```python
from build123d import *

# Parameters (mm, degrees)
CUT_EXTRUDE1_DEPTH      = 8.470943715
CUT_EXTRUDE1_DEPTH_BACK = 8.470943715
SKETCH3_OUTSIDE_W       = 10.214
SKETCH3_OUTSIDE_H       = 10.214
SKETCH3_OUTSIDE_W_2     = 4
SKETCH3_OUTSIDE_H_2     = 5
CUT_EXTRUDE2_DEPTH      = 7.641159537
CUT_EXTRUDE2_DEPTH_BACK = 7.641159537
SKETCH4_OUTSIDE_W       = 9.868
SKETCH4_OUTSIDE_H       = 8.768
SKETCH4_OUTSIDE_W_2     = 5
SKETCH4_OUTSIDE_H_2     = 5
SKETCH5_R               = 0.75
BOSS_EXTRUDE1_DEPTH     = 1.5
SKETCH6_R               = 1.5
BOSS_EXTRUDE2_DEPTH     = 2


with BuildPart() as part:
    # Sketch2 → Revolve3 (revolve)
    with BuildSketch(Plane(origin=(0, 0, 0), x_dir=(0, 0, -1), z_dir=(1, 0, 0))):
        with BuildLine():
            Line((0, 0), (0, 6.1))
            ThreePointArc((0, 6.1), (3.05, 3.05), (0, 0))
        make_face()
    revolve(axis=Axis((0, 0, 0), (0, 1, 0)))

    # Sketch3 outside → Cut-Extrude1 (cut, two sides: drawn at the far end of the back side and taken through both)
    with BuildSketch(Plane(origin=(0, 0, 0), x_dir=(0, 0, -1), z_dir=(1, 0, 0)).offset(-CUT_EXTRUDE1_DEPTH_BACK)):
        with Locations((0, 3.05)):
            Rectangle(SKETCH3_OUTSIDE_W, SKETCH3_OUTSIDE_H)
        with Locations((0, 3.05)):
            Rectangle(SKETCH3_OUTSIDE_W_2, SKETCH3_OUTSIDE_H_2, mode=Mode.SUBTRACT)
    extrude(amount=CUT_EXTRUDE1_DEPTH + CUT_EXTRUDE1_DEPTH_BACK, mode=Mode.SUBTRACT)

    # Sketch4 outside → Cut-Extrude2 (cut, two sides: drawn at the far end of the back side and taken through both)
    with BuildSketch(Plane.XY.offset(-CUT_EXTRUDE2_DEPTH_BACK)):
        with Locations((0, 3.05)):
            Rectangle(SKETCH4_OUTSIDE_W, SKETCH4_OUTSIDE_H)
        with Locations((0, 3.05)):
            Rectangle(SKETCH4_OUTSIDE_W_2, SKETCH4_OUTSIDE_H_2, mode=Mode.SUBTRACT)
    extrude(amount=CUT_EXTRUDE2_DEPTH + CUT_EXTRUDE2_DEPTH_BACK, mode=Mode.SUBTRACT)

    # Sketch5 → Boss-Extrude1 (add)
    with BuildSketch(Plane(origin=(2.5, 0, 0), x_dir=(0, 0, -1), z_dir=(1, 0, 0))):
        with Locations((0, 3.05)):
            Circle(SKETCH5_R)
    boss_extrude1 = extrude(amount=BOSS_EXTRUDE1_DEPTH)

    # Mirror1: Boss-Extrude1 across plane
    add(boss_extrude1.mirror(Plane(origin=(0, 0, 0), x_dir=(0, 0, 1), z_dir=(1, 0, 0))))

    # Sketch6 → Boss-Extrude2 (add)
    with BuildSketch(Plane(origin=(0, 0, -2), x_dir=(-1, 0, 0), z_dir=(0, 0, -1))):
        with Locations(Location((0, 3.05, 0), (0, 0, 90))):
            Circle(SKETCH6_R)
    boss_extrude2 = extrude(amount=BOSS_EXTRUDE2_DEPTH)

    # Mirror2: Boss-Extrude2 across plane
    add(boss_extrude2.mirror(Plane.XY))


solid = part.part
```
Design review of the part built by this model. Coordinates are the model's own, in mm. A direction names the side the tool comes from. Give positions to 0.01 mm unless a question says otherwise; leave off trailing zeros. Write each loop counter-clockwise with the first axis right and the second up, starting at its lowest first coordinate (ties: lowest second). Pieces come first, ordered by that corner, then holes. Notation, with made-up numbers: (75, -37) - (114, -37) arc R14 cw to (114, -30) - close; hole circle Ø8 at (-30.5, 22). An arc over 180 degrees is marked (long way). Return JSON: item names as keys, results as strings. Group by question number.
(1) We need section A-A, the plane y = 3.05. Give the boundary of the cut face in (x, z), then the cut area to 3 significant figures.
(2) Insertion check: pin 1 (1.5 mm diameter, centred on y = 4.5, z = 2, fed in from +X); pin 2 (1 mm diameter, centred on y = 4.5, z = 2, fed in from +X); pin 3 (1.5 mm diameter, centred on y = 3.5, z = 1.5, fed in from -X). Each pin has a flat end and moves straight along its axis. Give the tip position at first contact, or say it passes through.
(3) We need section D-D, the plane z = -2.25. Give the boundary of the cut face in (x, y), then the cut area to 3 significant figures.
(4) Mouldability with a two-part tool opening along Y and no side actions: class faces 4 (the cylindrical face through (3.24, 2.318, 0.163)), 5 (the flat face through (0, 0.55, 0)), 6 (the flat face through (0, 3, 4)) as +Y half, -Y half, draft (parallel to the pull), parting line (faces both ways), or undercut.
(5) We need section C-C, the plane z = 0. Give the boundary of the cut face in (x, y), then the cut area to 3 significant figures.
(6) Machinability: for faces 1 (the flat face through (-2.5, 3, 1)), 2 (the flat face through (0, 5, 2)), 3 (the cylindrical face through (0.45, 4.48, -2.99)), which of the approach directions +Z, -Z, +X, -X, +Y, -Y give a long, thin tool a straight path to every point of the face, cutting with its end or side? Answer none if there is none.
(7) To check wall thickness, follow probe 1 along Z at (x, y) = (1.75, 2.45); probe 2 along X at (y, z) = (1.5, 0.75); probe 3 along X at (y, z) = (3.15, -3). State the ranges of each line that lie inside material, in increasing order.
(8) We need section B-B, the plane x = 0. Give the boundary of the cut face in (y, z).
Reported:
{
 "1": {"outline": "(-4, -0.75) - (-2.5, -0.75) - (-2.5, -1.75) arc R3.05 ccw to (-2.3, -2) - (-1.5, -2) - (-1.5, -4) - (1.5, -4) - (1.5, -2) - (2.3, -2) arc R3.05 ccw to (2.5, -1.75) - (2.5, -0.75) - (4, -0.75) - (4, 0.75) - (2.5, 0.75) - (2.5, 1.75) arc R3.05 ccw to (2.3, 2) - (1.5, 2) - (1.5, 4) - (-1.5, 4) - (-1.5, 2) - (-2.3, 2) arc R3.05 ccw to (-2.5, 1.75) - (-2.5, 0.75) - (-4, 0.75) - close", "area": "36.4 mm2"},
 "2": {"pin 1": "stops at x = 2.5", "pin 2": "stops at x = 2.33", "pin 3": "stops at x = -2.5"},
 "3": {"outline": "circle Ø3 at (0, 3.05)", "area": "7.07 mm2"},
 "4": {"face 4": "parting line", "face 5": "-Y half", "face 6": "draft"},
 "5": {"outline": "(-4, 2.3) - (-2.5, 2.3) - (-2.5, 1.3) arc R3.05 ccw to (-1.75, 0.55) - (1.75, 0.55) arc R3.05 ccw to (2.5, 1.3) - (2.5, 2.3) - (4, 2.3) - (4, 3.8) - (2.5, 3.8) - (2.5, 4.8) arc R3.05 ccw to (1.75, 5.55) - (-1.75, 5.55) arc R3.05 ccw to (-2.5, 4.8) - (-2.5, 3.8) - (-4, 3.8) - close", "area": "28.5 mm2"},
 "6": {"face 1": "-X", "face 2": "+Z", "face 3": "-Z"},
 "7": {"probe 1": "z = -2 to 2", "probe 2": "x = -2.5 to 2.5", "probe 3": "x = -1.5 to 1.5"},
 "8": {"outline": "(0.55, -1.75) arc R3.05 ccw to (0.75, -2) - (1.55, -2) - (1.55, -4) - (4.55, -4) - (4.55, -2) - (5.35, -2) arc R3.05 ccw to (5.55, -1.75) - (5.55, 1.75) arc R3.05 ccw to (5.35, 2) - (4.55, 2) - (4.55, 4) - (1.55, 4) - (1.55, 2) - (0.75, 2) arc R3.05 ccw to (0.55, 1.75) - close"}
}
